Source: CAD feature listing. Evaluate the final solid. Frame: model axes, mm. A direction names the side the tool comes from. Coordinates: 2 decimals unless noted, no trailing zeros. Loops run counter-clockwise (first coordinate to the right, second up) from the corner with the lowest first, then second, coordinate; pieces in that order, holes last. Notation, with made-up numbers: (18.5, 82.5) -> (37.5, 82.5) arc R33 cw to (37.5, 119.5) -> close; hole circle Ø11 at (-29, -10.75). An arc over 180 degrees is marked (long way). Answer as a JSON object with one key per item and string values. Group by question number.
from build123d import *

# Parameters (mm, degrees)
SKETCH_236_R                = 3
EXTRUDE_290_DEPTH           = 115
HOLE_WIZARD_M41_D           = 3.3
HOLE_WIZARD_M41_DEPTH       = 12
HOLE_WIZARD_M41_CSINK_D     = 4.5
HOLE_WIZARD_M41_CSINK_ANGLE = 90
HOLE_WIZARD_M41_TIP         = 0.991420021
HOLE_WIZARD_M42_D           = 3.3
HOLE_WIZARD_M42_DEPTH       = 12
HOLE_WIZARD_M42_CSINK_D     = 4.5
HOLE_WIZARD_M42_CSINK_ANGLE = 90
HOLE_WIZARD_M42_TIP         = 0.991420021
CHAMFER_1_SIZE              = 0.3


with BuildPart() as part:
    # Sketch 236 → Extrude 290 (new body)
    with BuildSketch(Plane.XY):
        Circle(SKETCH_236_R)
    extrude(amount=EXTRUDE_290_DEPTH)

    # Отверстие обработанное метчиком M41
    with Locations(Plane.XY.offset(115)):
        with Locations((0, 0)):
            CounterSinkHole(HOLE_WIZARD_M41_D / 2, HOLE_WIZARD_M41_CSINK_D / 2, depth=HOLE_WIZARD_M41_DEPTH, counter_sink_angle=HOLE_WIZARD_M41_CSINK_ANGLE)
            with Locations((0, 0, -(HOLE_WIZARD_M41_DEPTH + HOLE_WIZARD_M41_TIP / 2))):  # 118° drill point
                Cone(0, HOLE_WIZARD_M41_D / 2, HOLE_WIZARD_M41_TIP, mode=Mode.SUBTRACT)

    # Отверстие обработанное метчиком M42
    with Locations(Plane(origin=(0, 0, 0), x_dir=(-1, 0, 0), z_dir=(0, 0, -1))):
        with Locations((0, 0)):
            CounterSinkHole(HOLE_WIZARD_M42_D / 2, HOLE_WIZARD_M42_CSINK_D / 2, depth=HOLE_WIZARD_M42_DEPTH, counter_sink_angle=HOLE_WIZARD_M42_CSINK_ANGLE)
            with Locations((0, 0, -(HOLE_WIZARD_M42_DEPTH + HOLE_WIZARD_M42_TIP / 2))):  # 118° drill point
                Cone(0, HOLE_WIZARD_M42_D / 2, HOLE_WIZARD_M42_TIP, mode=Mode.SUBTRACT)

    # Фаска1
    chamfer_1_edges = [part.edges().sort_by_distance(p)[0] for p in [
        (-3, 0, 0),
        (-3, 0, 115),
    ]]
    chamfer(chamfer_1_edges, length=CHAMFER_1_SIZE)


solid = part.part
1. Reachability of faces 1 (the face through (-1.216, 1.115, 6.38)), 2 (the face through (1.216, 1.115, 108.62)) from +Z, -Z, +X, -X, +Y, -Y: full face, straight path, thin tool, end or side. Return the list, or none.
2. Pin query (flat end, axial travel): pin 1 Ø1 at (x, z) = (-2, 75.5) entering from +Y; pin 2 Ø2 at (x, y) = (0, 0) entering from +Z; pin 3 Ø2 at (x, z) = (-2, 26) entering from +Y. Return the tip coordinate at first contact, or that it passes through.
3. Section query A-A on z = 17. Return loops of the section in (x, y), then the cut area to 3 significant figures.
4. Mould query, pull axis X, two halves, no side actions, for faces 3 (the face through (-3, 0, 57)), 4 (the face through (0.1, -0.3, 12.8)), 5 (the face through (-0.1, -0.3, 102.2)). Classes: pulls with the +X half, pulls with the -X half, needs draft (parallel to the pull), parting line crosses it, or undercut.
5. Ray query, L1, parallel to Y at x = 0, z = 111; L2, parallel to Y at x = 0.7, z = 5; L3, parallel to Y at x = -2.5, z = 102.5. Return the intervals inside material, ascending.
Solved:
{
 "1": {"face 1": "-Z", "face 2": "+Z"},
 "2": {"pin 1": "y = 2.6", "pin 2": "z = 102.61", "pin 3": "y = 2.83"},
 "3": {"outline": "circle Ø6 at (0, 0)", "area": "28.3 mm^2"},
 "4": {"face 3": "parting line crosses it", "face 4": "undercut", "face 5": "undercut"},
 "5": {"L1": "-3 to -1.65, 1.65 to 3", "L2": "-2.92 to -1.49, 1.49 to 2.92", "L3": "-1.66 to 1.66"}
}
